from build123d import *

# Parameters (mm, degrees)
SKETCH1_R           = 1.905
BOSS_EXTRUDE1_DEPTH = 4.7625
CUT_EXTRUDE3_DEPTH  = 5.7625


with BuildPart() as part:
    # Sketch1 → Boss-Extrude1 (new body)
    with BuildSketch(Plane(origin=(0, 0, 0), x_dir=(1, 0, 0), z_dir=(0, 1, 0))):
        with BuildLine():
            ThreePointArc((0, 176.53), (1.859871939, 181.020128061), (6.35, 182.88))
            Line((6.35, 182.88), (87.63, 182.88))
            ThreePointArc((87.63, 182.88), (92.120128061, 181.020128061), (93.98, 176.53))
            Line((93.98, 176.53), (93.98, 6.35))
            ThreePointArc((93.98, 6.35), (92.120128061, 1.859871939), (87.63, 0))
            Line((87.63, 0), (6.35, 0))
            ThreePointArc((6.35, 0), (1.859871939, 1.859871939), (0, 6.35))
            Line((0, 6.35), (0, 176.53))
        make_face()
        with Locations(Location((90.324076836, 3.655923164, 0), (0, 0, 270))):  # turned: the seam where the file's is
            Circle(SKETCH1_R, mode=Mode.SUBTRACT)
        with Locations(Location((3.655923164, 3.655923164, 0), (0, 0, 270))):  # turned: the seam where the file's is
            Circle(SKETCH1_R, mode=Mode.SUBTRACT)
        with Locations(Location((90.324076836, 179.224076836, 0), (0, 0, 270))):  # turned: the seam where the file's is
            Circle(SKETCH1_R, mode=Mode.SUBTRACT)
        with Locations(Location((3.655923164, 179.224076836, 0), (0, 0, 270))):  # turned: the seam where the file's is
            Circle(SKETCH1_R, mode=Mode.SUBTRACT)
    extrude(amount=BOSS_EXTRUDE1_DEPTH)

    # Sketch2 → Cut-Extrude3 (cut, through all)
    with BuildSketch(Plane(origin=(0, 0, 0), x_dir=(1, 0, 0), z_dir=(0, 1, 0))):
        Polygon((44.330866221, 142.412423135), (55.583348796, 112.48561291), (50.236412259, 113.523076227), (49.358559843, 90.619091365), (51.892366687, 90.359727043), (57.897684242, 88.783579573), (66.03778893, 104.904168998), (61.089973403, 107.29831442), (81.200790115, 119.747856132), (61.568701793, 78.568503007), (58.865309307, 80.004989053), (55.003504896, 81.127248207), (49.039350105, 81.92031082), (47.602864059, 16.00137357), (44.330866221, 16.001385635), (41.058234971, 16.001385635), (39.621748925, 81.920322885), (33.691252468, 81.127263288), (29.825707906, 80.005004135), (27.092397237, 78.568515072), (7.62, 119.747868197), (27.730816712, 107.298326485), (22.6233101, 104.904181063), (30.763414788, 88.783591638), (36.738802094, 90.359739108), (39.302539188, 90.61910343), (38.424686771, 113.523088292), (33.077750234, 112.485624975), align=None)
    extrude(amount=CUT_EXTRUDE3_DEPTH, mode=Mode.SUBTRACT)


solid = part.part
Read the model definition and answer for the solid it produces. Units are mm, in the model's axes. A direction names the side the tool comes from. Give positions to 0.01 mm unless a question says otherwise; leave off trailing zeros. Write each loop counter-clockwise with the first axis right and the second up, starting at its lowest first coordinate (ties: lowest second). Pieces come first, ordered by that corner, then holes. Notation, with made-up numbers: (78, -5) - (82, -5) arc R16 cw to (82, 23) - close; hole circle Ø1 at (53.25, 10.25). An arc over 180 degrees is marked (long way). Answer in a Markdown table with one row per item. Add a question column.
Item 1: Section B-B, the plane x = 74 is taken. Write down the section's boundary in (y, z), and give its area (3 significant figures).
Item 2: A tool of negligible diameter and unlimited length cuts with its end or side. For faces 1 (the face through (49.878, 2.348, -127.659)), 2 (the face through (1.91, 2.35, -1.81)), from which of +Z, -Z, +X, -X, +Y, -Y can it reach the whole face along a straight path? Write none if from no direction.
Item 3: Section C-C, the plane z = -94.5 is taken. Write down the section's boundary in (x, y), and give its area (3 significant figures).
Item 4: A flat-ended cylindrical pin translates along its axis: P1, Ø1.5, axis at x = 68.5, z = -156.5, coming from the -Y side. Find the tip coordinate at first contact, or state that the pin passes through.
Item 5: Determine the mould class of faces 3 (the face through (1.81, 2.35, -180.97)), 4 (the face through (52.947, 2.348, -112.997)), 5 (the face through (92.17, 2.35, -1.91)), 6 (the face through (58, 4.762, -93)) for opening direction Z: pulls with the +Z half, pulls with the -Z half, needs draft (parallel to the pull), parting line crosses it, or undercut.
Item 6: Section A-A, the plane z = -29.5 is taken. Write down the section's boundary in (x, y), and give its area (3 significant figures).
Item 7: Section D-D, the plane y = 3.9 is taken. Count the separate pieces of the cut face and the enclosed holes in it, and give its area (3 significant figures).
Item 8: Find the intervals of material crossed by L1, parallel to X at y = 0.55, z = -106; L2, parallel to X at y = 4.5, z = -95; L3, parallel to X at y = 2.65, z = -60.5, in increasing order.
Recorded:
| question | item | result |
|---|---|---|
| 1 | outline | (0, -182.88) - (4.76, -182.88) - (4.76, -115.29) - (0, -115.29) - close; (0, -104.64) - (4.76, -104.64) - (4.76, 0) - (0, 0) - close |
| 1 | area | 820 mm2 |
| 2 | face 1 | +Y, -Y |
| 2 | face 2 | +Z, -X, +Y, -Y |
| 3 | outline | (0, 0) - (19.56, 0) - (19.56, 4.76) - (0, 4.76) - close; (27.88, 0) - (39.15, 0) - (39.15, 4.76) - (27.88, 4.76) - close; (49.51, 0) - (60.78, 0) - (60.78, 4.76) - (49.51, 4.76) - close; (69.16, 0) - (93.98, 0) - (93.98, 4.76) - (69.16, 4.76) - close |
| 3 | area | 319 mm2 |
| 4 | P1 | stops at y = 0 |
| 5 | face 3 | pulls with the -Z half |
| 5 | face 4 | undercut |
| 5 | face 5 | pulls with the +Z half |
| 5 | face 6 | needs draft |
| 6 | outline | (0, 0) - (40.76, 0) - (40.76, 4.76) - (0, 4.76) - close; (47.9, 0) - (93.98, 0) - (93.98, 4.76) - (47.9, 4.76) - close |
| 6 | area | 414 mm2 |
| 7 | separate pieces | 1 |
| 7 | enclosed holes | 5 |
| 7 | area | 15,200 mm2 |
| 8 | L1 | x = 0 to 14.12, 24.96 to 38.71, 49.95 to 63.77, 74.65 to 93.98 |
| 8 | L2 | x = 0 to 19.32, 27.62 to 39.13, 49.53 to 61.04, 69.4 to 93.98 |
| 8 | L3 | x = 0 to 40.09, 48.57 to 93.98 |
